Input: part model. Units: mm. Frame: model coordinates. A direction names the side the tool comes from. Coordinates: 2 decimals unless noted, no trailing zeros. Write each loop counter-clockwise with the first axis right and the second up, starting at its lowest first coordinate (ties: lowest second). Pieces come first, ordered by that corner, then holes.
from build123d import *

# Parameters (mm, degrees)
ESTRUSIONE_ESTRUSIONE1_DEPTH  = 10
TAGLIO_ESTRUSIONE1_DEPTH      = 3
SCHIZZO4_W                    = 80
SCHIZZO4_H                    = 5
ESTRUSIONE_ESTRUSIONE2_DEPTH  = 35
ESTRUSIONE_ESTRUSIONE4_DEPTH  = 80
SCHIZZO7_W                    = 80
SCHIZZO7_H                    = 5
ESTRUSIONE_ESTRUSIONE5_DEPTH  = 7
TAGLIO_ESTRUSIONE2_REACH      = 112.369
SCHIZZO8_R                    = 1.5
RACCORDO1_R                   = 5
RACCORDO2_R                   = 5
TAGLIO_ESTRUSIONE3_DEPTH      = 111.368700273
TAGLIO_ESTRUSIONE3_DEPTH_BACK = 10
SCHIZZO11_R                   = 4
TAGLIO_ESTRUSIONE4_DEPTH      = 3
SCHIZZO12_W                   = 12
SCHIZZO12_H                   = 12
ESTRUSIONE_ESTRUSIONE6_DEPTH  = 40
SCHIZZO13_R                   = 1.5
TAGLIO_ESTRUSIONE5_DEPTH      = 111.368700273
SCHIZZO14_R                   = 4
TAGLIO_ESTRUSIONE6_DEPTH      = 10


with BuildPart() as part:
    # Schizzo1 → Estrusione-Estrusione1 (new body)
    with BuildSketch(Plane.XY):
        with BuildLine():
            Line((-76.016095604, 20), (76.016095604, 20))
            ThreePointArc((76.016095604, 20), (92.5, 0), (76.016095604, -20))
            Line((76.016095604, -20), (-76.016095604, -20))
            ThreePointArc((-76.016095604, -20), (-92.5, 0), (-76.016095604, 20))
        make_face()
    extrude(amount=ESTRUSIONE_ESTRUSIONE1_DEPTH)

    # Schizzo3 → Taglio-Estrusione1 (cut)
    with BuildSketch(Plane.XY.offset(10)):
        with BuildLine():
            Line((-75.5, -15), (75.5, -15))
            ThreePointArc((75.5, -15), (87.5, 0), (75.5, 15))
            Line((75.5, 15), (-75.5, 15))
            ThreePointArc((-75.5, 15), (-87.5, 0), (-75.5, -15))
        make_face()
    extrude(amount=-TAGLIO_ESTRUSIONE1_DEPTH, mode=Mode.SUBTRACT)

    # Schizzo4 → Estrusione-Estrusione2 (add)
    with BuildSketch(Plane.XY.offset(10)):
        with Locations((0, -17.5)):
            Rectangle(SCHIZZO4_W, SCHIZZO4_H)
    estrusione_estrusione2 = extrude(amount=ESTRUSIONE_ESTRUSIONE2_DEPTH)

    # Schizzo6 → Estrusione-Estrusione4 (add)
    with BuildSketch(Plane(origin=(40, 0, 0), x_dir=(0, 0, -1), z_dir=(1, 0, 0))):
        Polygon((-40, -15), (-40, -12.81), (-7, -15), align=None)
    estrusione_estrusione4 = extrude(amount=-ESTRUSIONE_ESTRUSIONE4_DEPTH)

    # Schizzo7 → Estrusione-Estrusione5 (add)
    with BuildSketch(Plane(origin=(0, -15, 0), x_dir=(1, 0, 0), z_dir=(0, 1, 0))):
        with Locations((0, -42.5)):
            Rectangle(SCHIZZO7_W, SCHIZZO7_H)
    estrusione_estrusione5 = extrude(amount=ESTRUSIONE_ESTRUSIONE5_DEPTH)

    # Taglio-Estrusione2: up to this plane
    taglio_estrusione2_end = Plane(origin=(-40, -12.81, 40), z_dir=(1.4576135341627736e-15, 0.9978051809344605, -0.0662179801892863))
    # Schizzo8 → Taglio-Estrusione2 (cut, up to the surface)
    with BuildSketch(Plane.XZ.offset(20), mode=Mode.PRIVATE) as taglio_estrusione2_sk1:
        with Locations(Location((-30, 13, 0), (0, 0, 270))):
            Circle(SCHIZZO8_R)
    taglio_estrusione2_tool1 = split(extrude(taglio_estrusione2_sk1.sketch, amount=-TAGLIO_ESTRUSIONE2_REACH, mode=Mode.PRIVATE), bisect_by=taglio_estrusione2_end, keep=Keep.BOTH, mode=Mode.PRIVATE)
    add(taglio_estrusione2_tool1.solids().sort_by_distance((-30, -20, 13))[0], mode=Mode.SUBTRACT)
    # Schizzo8 → Taglio-Estrusione2 (cut, up to the surface)
    with BuildSketch(Plane.XZ.offset(20), mode=Mode.PRIVATE) as taglio_estrusione2_sk2:
        with Locations(Location((-30, 32, 0), (0, 0, 270))):
            Circle(SCHIZZO8_R)
    taglio_estrusione2_tool2 = split(extrude(taglio_estrusione2_sk2.sketch, amount=-TAGLIO_ESTRUSIONE2_REACH, mode=Mode.PRIVATE), bisect_by=taglio_estrusione2_end, keep=Keep.BOTH, mode=Mode.PRIVATE)
    add(taglio_estrusione2_tool2.solids().sort_by_distance((-30, -20, 32))[0], mode=Mode.SUBTRACT)
    # Schizzo8 → Taglio-Estrusione2 (cut, up to the surface)
    with BuildSketch(Plane.XZ.offset(20), mode=Mode.PRIVATE) as taglio_estrusione2_sk3:
        with Locations(Location((30, 13, 0), (0, 0, 270))):
            Circle(SCHIZZO8_R)
    taglio_estrusione2_tool3 = split(extrude(taglio_estrusione2_sk3.sketch, amount=-TAGLIO_ESTRUSIONE2_REACH, mode=Mode.PRIVATE), bisect_by=taglio_estrusione2_end, keep=Keep.BOTH, mode=Mode.PRIVATE)
    add(taglio_estrusione2_tool3.solids().sort_by_distance((30, -20, 13))[0], mode=Mode.SUBTRACT)
    # Schizzo8 → Taglio-Estrusione2 (cut, up to the surface)
    with BuildSketch(Plane.XZ.offset(20), mode=Mode.PRIVATE) as taglio_estrusione2_sk4:
        with Locations(Location((30, 32, 0), (0, 0, 270))):
            Circle(SCHIZZO8_R)
    taglio_estrusione2_tool4 = split(extrude(taglio_estrusione2_sk4.sketch, amount=-TAGLIO_ESTRUSIONE2_REACH, mode=Mode.PRIVATE), bisect_by=taglio_estrusione2_end, keep=Keep.BOTH, mode=Mode.PRIVATE)
    add(taglio_estrusione2_tool4.solids().sort_by_distance((30, -20, 32))[0], mode=Mode.SUBTRACT)

    # Specchia1: Estrusione-Estrusione2, Estrusione-Estrusione4, Estrusione-Estrusione5 across plane
    add(estrusione_estrusione2.mirror(Plane.ZX))
    add(estrusione_estrusione4.mirror(Plane.ZX))
    add(estrusione_estrusione5.mirror(Plane.ZX))

    # Raccordo1
    raccordo1_edges = [part.edges().sort_by_distance(p)[0] for p in [
        (0, -20, 45),
    ]]
    fillet(raccordo1_edges, radius=RACCORDO1_R)

    # Raccordo2
    raccordo2_edges = [part.edges().sort_by_distance(p)[0] for p in [
        (0, 20, 45),
    ]]
    fillet(raccordo2_edges, radius=RACCORDO2_R)

    # Schizzo9 → Taglio-Estrusione3 (cut, two sides)
    with BuildSketch(Plane.XZ.offset(20)) as taglio_estrusione3_sk:
        Polygon((-4, 11), (-4, 3), (4, 3), (4, 11), (10, 11), (10, 31), (-10, 31), (-10, 11), align=None)
    extrude(amount=TAGLIO_ESTRUSIONE3_DEPTH, mode=Mode.SUBTRACT)
    extrude(taglio_estrusione3_sk.sketch, amount=-TAGLIO_ESTRUSIONE3_DEPTH_BACK, mode=Mode.SUBTRACT)

    # Schizzo11 → Taglio-Estrusione4 (cut)
    with BuildSketch(Plane(origin=(0, -15.396736192, 1.021783402), x_dir=(1, 0, 0), z_dir=(1.4576135341627738e-15, 0.9978051809344605, -0.06621798018928632))):
        with Locations(Location((-30, -12.004564445, 0), (0, 0, 270))):
            Circle(SCHIZZO11_R)
        with Locations(Location((-30, -31.046357736, 0), (0, 0, 270))):
            Circle(SCHIZZO11_R)
        with Locations(Location((30, -31.046357736, 0), (0, 0, 270))):
            Circle(SCHIZZO11_R)
        with Locations(Location((30, -12.004564445, 0), (0, 0, 270))):
            Circle(SCHIZZO11_R)
    extrude(amount=-TAGLIO_ESTRUSIONE4_DEPTH, mode=Mode.SUBTRACT)

    # Schizzo12 → Estrusione-Estrusione6 (add)
    with BuildSketch(Plane.XZ.offset(20)):
        with Locations((70.016095604, -6)):
            Rectangle(SCHIZZO12_W, SCHIZZO12_H)
        with Locations((-70.016095604, -6)):
            Rectangle(SCHIZZO12_W, SCHIZZO12_H)
        with Locations((0, -6)):
            Rectangle(SCHIZZO12_W, SCHIZZO12_H)
    extrude(amount=-ESTRUSIONE_ESTRUSIONE6_DEPTH)

    # Schizzo13 → Taglio-Estrusione5 (cut, through all)
    with BuildSketch(Plane.XZ.offset(20)):
        with Locations(Location((-70.016095604, -6, 0), (0, 0, 270))):
            Circle(SCHIZZO13_R)
        with Locations(Location((0, -6, 0), (0, 0, 270))):
            Circle(SCHIZZO13_R)
        with Locations(Location((70.016095604, -6, 0), (0, 0, 270))):
            Circle(SCHIZZO13_R)
    extrude(amount=-TAGLIO_ESTRUSIONE5_DEPTH, mode=Mode.SUBTRACT)

    # Schizzo14 → Taglio-Estrusione6 (cut)
    with BuildSketch(Plane.XZ.offset(20)):
        with Locations(Location((-70.016095604, -6, 0), (0, 0, 270))):
            Circle(SCHIZZO14_R)
        with Locations(Location((0, -6, 0), (0, 0, 270))):
            Circle(SCHIZZO14_R)
        with Locations(Location((70.016095604, -6, 0), (0, 0, 270))):
            Circle(SCHIZZO14_R)
    taglio_estrusione6 = extrude(amount=-TAGLIO_ESTRUSIONE6_DEPTH, mode=Mode.SUBTRACT)

    # Specchia2: Taglio-Estrusione6 across plane
    add(taglio_estrusione6.mirror(Plane.ZX), mode=Mode.SUBTRACT)

    # TaglioSuperficie1
    split(bisect_by=Plane(origin=(0, 0, 0), x_dir=(1, 0, 0), z_dir=(0, 1, 0)), keep=Keep.TOP)


solid = part.part
Item 1: Section query C-C, the plane z = 14. Return loops of the section in (x, y), then the cut area to 3 significant figures.
Item 2: Section query B-B, the plane z = 4. Return loops of the section in (x, y) (3 decimals), then the cut area to 3 significant figures.
Item 3: Access query for faces 4 (the face through (-58, 15, 9)), 5 (the face through (-1, 8, 42)), 6 (the face through (6, 10, -6)). Directions: +Z, -Z, +X, -X, +Y, -Y. A direction counts if a zero-diameter tool reaches every point of the face in a straight line with its end or side. Return the directions, or none.
Item 4: Pin query (flat end, axial travel): pin 1 Ø6 at (x, y) = (19, 3.5) entering from +Z; pin 2 Ø12 at (x, y) = (9, 4.5) entering from +Z; pin 3 Ø3.5 at (x, z) = (63.5, 9) entering from -Y; pin 4 Ø5 at (x, y) = (-32, 12.5) entering from -Z. Return the tip coordinate at first contact, or that it passes through.
Item 5: Section query A-A, the plane x = -54.5. Return loops of the section in (y, z).
Item 6: Material intervals for line 1 (X direction, y = 14.5, z = -6); line 2 (X direction, y = 2.75, z = -9.5); line 3 (Z direction, x = -39, y = 9.75), sorted ascending.
Item 7: Pull-direction query (Z, two-part tool) for faces 1 (the face through (71.28, 4.93, -6.81)), 2 (the face through (-40, 17, 30)), 3 (the face through (-68, 16, 10)); classes: released by +Z, released by -Z, zero draft, split by the parting line, or undercut.
The answers:
1. outline: (-40, 14.54) - (40, 14.54) - (40, 20) - (-40, 20) - close
1. area: 437 mm2
2. outline: (-92.5, 0) - (92.5, 0) arc R20.375 ccw to (76.016, 20) - (-76.016, 20) arc R20.375 ccw to start
2. area: 3,540 mm2
3. face 4: +Z, -Y
3. face 5: +Z, +X, -X, -Y
3. face 6: -Z, +Y, -Y
4. pin 1: stops at z = 7
4. pin 2: stops at z = 45
4. pin 3: stops at y = 15
4. pin 4: stops at z = 0
5. outline: (0, 0) - (20, 0) - (20, 10) - (15, 10) - (15, 7) - (0, 7) - close
6. line 1: x = -76.02 to -74.02, -66.02 to -64.02, -6 to -4, 4 to 6, 64.02 to 66.02, 74.02 to 76.02
6. line 2: x = -76.02 to -64.02, -6 to 6, 64.02 to 76.02
6. line 3: z = 0 to 7, 40 to 45
7. face 1: undercut
7. face 2: zero draft
7. face 3: released by +Z
